Check sheet for the modelled part. Datum: model origin and axes. Units: mm. Face numbers are marked on the shaded views. A direction names the side the tool comes from. Give positions to 0.01 mm unless a question says otherwise; leave off trailing zeros. Order: outer loops, then holes, each group sorted by start corner. A loop starts at its lowest first (then second) coordinate and runs counter-clockwise, first axis right, second up.
Item 1: Release check for a two-part mould opening along X. For the marked faces 5, 6 and 7 record: released by +X, released by -X, zero draft, split by the parting line, or undercut.
Item 2: Access from +Z, -Z, +X, -X, +Y, -Y to the whole of each face (thin tool, end or side, straight path). Record for the marked faces 1, 2, 3 and 4.
Item 3: Sectioned sample at D-D on y = 120. Record the boundary of the cut face in (x, z), and give its area (3 significant figures).
Item 4: Gauge pin test, flat ends, axial feed: P1, Ø1.5, axis at y = 134.5, z = -1, coming from the -X side; P2, Ø2, axis at x = -8.5, z = 7, coming from the +Y side; P3, Ø6, axis at x = 10, y = 80.5, coming from the -Z side; P4, Ø11, axis at x = 0, y = 120, coming from the +Z side. Record the tip position at first contact, or that the pin passes through.
Item 5: Sectioned sample at A-A on x = 0. Record the boundary of the cut face in (y, z).
Item 6: Sectioned sample at C-C on z = 7.5. Record the boundary of the cut face in (x, y), and give its area (3 significant figures).
Item 7: Sectioned sample at B-B on y = 0. Record the boundary of the cut face in (x, z).
Item 8: Material ranges on line 1 along Y through (x, z) = (0, -2.5); line 2 along X through (y, z) = (-0.5, -3.75); line 3 along Z through (x, y) = (-7, 39), recorded low to high.
from build123d import *

# Parameters (mm, degrees)
SKETCH1_R             = 21
SKETCH1_R_2           = 16
BOSS_EXTRUDE1_DEPTH   = 10
SKETCH1_R_3           = 12.5
SKETCH1_R_4           = 6.25
BOSS_EXTRUDE1_2_DEPTH = 10
BOSS_EXTRUDE2_DEPTH   = 6
CUT_EXTRUDE1_START    = 6
CUT_EXTRUDE1_DEPTH    = 16


with BuildPart() as part:
    # Sketch1 → Boss-Extrude1 (new body, symmetric)
    with BuildSketch(Plane.XY):
        Circle(SKETCH1_R)
        Circle(SKETCH1_R_2, mode=Mode.SUBTRACT)
    extrude(amount=BOSS_EXTRUDE1_DEPTH, both=True)



with BuildPart() as body_2:
    # Sketch1 → Boss-Extrude1 2 (new body, symmetric)
    with BuildSketch(Plane.XY):
        with Locations((0, 120)):
            Circle(SKETCH1_R_3)
        with Locations((0, 120)):
            Circle(SKETCH1_R_4, mode=Mode.SUBTRACT)
    extrude(amount=BOSS_EXTRUDE1_2_DEPTH, both=True)


with BuildPart() as part_1:
    add(part.part)

    add(body_2.part)  # Boss-Extrude2 merges body 2
    # Sketch1_3 → Boss-Extrude2 (add, symmetric)
    with BuildSketch(Plane.XY):
        with BuildLine():
            ThreePointArc((8, 110.395313644), (0, 107.5), (-8, 110.395313644))
            Line((-8, 110.395313644), (-8, 75.395313644))
            ThreePointArc((-8, 75.395313644), (-10.96842855, 40.709642053), (-19.787382488, 7.032744434))
            ThreePointArc((-19.787382488, 7.032744434), (0, 21), (19.787382488, 7.032744434))
            ThreePointArc((19.787382488, 7.032744434), (10.96842855, 40.709642053), (8, 75.395313644))
            Line((8, 75.395313644), (8, 110.395313644))
        make_face()
        with BuildLine():
            Line((-6.25, 135.825317547), (-6.25, 130.825317547))
            ThreePointArc((-6.25, 130.825317547), (0, 132.5), (6.25, 130.825317547))
            Line((6.25, 130.825317547), (6.25, 135.825317547))
            Line((6.25, 135.825317547), (-6.25, 135.825317547))
        make_face()
        with BuildLine():
            ThreePointArc((17, -12.328828006), (0, -21), (-17, -12.328828006))
            Line((-17, -12.328828006), (-17, -24.328828006))
            Line((-17, -24.328828006), (17, -24.328828006))
            Line((17, -24.328828006), (17, -12.328828006))
        make_face()
    extrude(amount=BOSS_EXTRUDE2_DEPTH, both=True)

    # Sketch2 → Cut-Extrude1 (cut, through all)
    with BuildSketch(Plane(origin=(0, 0, 0), x_dir=(0, 0, -1), z_dir=(1, 0, 0)).offset(CUT_EXTRUDE1_START)):
        with BuildLine():
            Line((-4, 100), (-4, 38))
            ThreePointArc((-4, 38), (0, 34), (4, 38))
            Line((4, 38), (4, 100))
            ThreePointArc((4, 100), (0, 104), (-4, 100))
        make_face()
    cut_extrude1 = extrude(amount=CUT_EXTRUDE1_DEPTH, mode=Mode.SUBTRACT)

    # Mirror1: Cut-Extrude1 across plane
    add(cut_extrude1.mirror(Plane(origin=(0, 0, 0), x_dir=(0, 0, 1), z_dir=(1, 0, 0))), mode=Mode.SUBTRACT)


solid = part_1.part
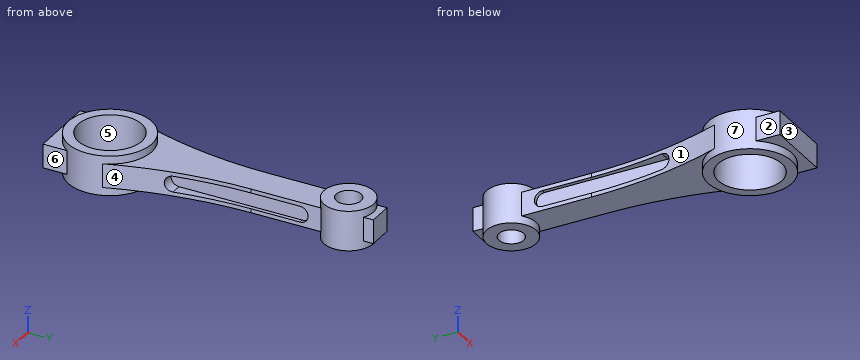
Report:
1. face 5: undercut
1. face 6: released by +X
1. face 7: split by the parting line
2. face 1: +Z, -Z, -X
2. face 2: +Z, -Z, -X, -Y
2. face 3: +Z, -Z, +X, -X, -Y
2. face 4: +Z, -Z, +X
3. outline: (-12.5, -10) - (-6.25, -10) - (-6.25, 10) - (-12.5, 10) - close; (6.25, -10) - (12.5, -10) - (12.5, 10) - (6.25, 10) - close
3. area: 250 mm2
4. P1: stops at x = -6.25
4. P2: stops at y = 130
4. P3: stops at z = -6
4. P4: passes through
5. outline: (-24.33, -6) - (-21, -6) - (-21, -10) - (-16, -10) - (-16, 10) - (-21, 10) - (-21, 6) - (-24.33, 6) - close; (16, -10) - (21, -10) - (21, -6) - (107.5, -6) - (107.5, -10) - (113.75, -10) - (113.75, 10) - (107.5, 10) - (107.5, 6) - (21, 6) - (21, 10) - (16, 10) - close; (126.25, -10) - (132.5, -10) - (132.5, -6) - (135.83, -6) - (135.83, 6) - (132.5, 6) - (132.5, 10) - (126.25, 10) - close
6. outline: circle Ø42 at (0, 0); circle Ø25 at (0, 120); hole circle Ø32 at (0, 0); hole circle Ø12.5 at (0, 120)
6. area: 949 mm2
7. outline: (-21, -10) - (-16, -10) - (-16, 10) - (-21, 10) - close; (16, -10) - (21, -10) - (21, 10) - (16, 10) - close
8. line 1: y = -24.33 to -16, 16 to 113.75, 126.25 to 135.83
8. line 2: x = -20.99 to -15.99, 15.99 to 20.99
8. line 3: z = -6 to -4, 4 to 6
